Geometry check sheet. Reference: the model listing, model coordinates, mm. Coordinates: 2 decimals unless noted, no trailing zeros. Order: outer loops, then holes, each group sorted by start corner. A loop starts at its lowest first (then second) coordinate and runs counter-clockwise, first axis right, second up. Notation, with made-up numbers: M 20,85.5 L 70,85.5 A26 ccw 70,118.5 Z; hole C 63.5,70 d6. An arc over 180 degrees is marked long. One line per item, written item: value. Start each with the question number.
1) Go/stop test with flat-tipped pins: P1, Ø6.5, axis at x = -45, z = -30.5, coming from the +Y side; P2, Ø1.6, axis at x = 61, y = 3.5, coming from the +Z side; P3, Ø5, axis at x = 28, z = 3.5, coming from the +Y side; P4, Ø1.9, axis at x = -60, y = 3, coming from the -Z side. Record where each tip stops, or that it passes through.
2) Thickness scan on L1, parallel to Z at x = -9, y = 0.45; L2, parallel to Z at x = 52.5, y = 2.5; L3, parallel to Z at x = 48.5, y = 2.5. Record the ranges inside material, lowest first. Write a range as from..to.
3) Sectioned sample at A-A, the plane z = 23.5. State how many separate pieces and enclosed holes the cut face has, then the cut area to 3 significant figures.
4) Sectioned sample at B-B, the plane x = 20. Enter the section's corners in (y, z), then the cut area to 3 significant figures.
```python
from build123d import *

# Parameters (mm, degrees)
SKETCH1_W           = 131.727
SKETCH1_H           = 90.551
SKETCH1_R           = 3.5
BOSS_EXTRUDE1_DEPTH = 10
SKETCH3_W           = 10
SKETCH3_H           = 10
BOSS_EXTRUDE3_DEPTH = 10
SKETCH4_R           = 3.15
CUT_EXTRUDE2_DEPTH  = 87.564320205
FILLET2_R           = 2.5
FILLET3_R           = 4
SKETCH5_R           = 4.975
CUT_EXTRUDE3_DEPTH  = 9.5


with BuildPart() as part:
    # Sketch1 → Boss-Extrude1 (new body)
    with BuildSketch(Plane(origin=(0, 0, 0), x_dir=(1, 0, 0), z_dir=(0, 1, 0))):
        Rectangle(SKETCH1_W, SKETCH1_H)
        with Locations(Location((-45, 30.5, 0), (0, 0, 270))):
            Circle(SKETCH1_R, mode=Mode.SUBTRACT)
        with Locations(Location((-27, 30.5, 0), (0, 0, 270))):
            Circle(SKETCH1_R, mode=Mode.SUBTRACT)
        with Locations(Location((-9, 30.5, 0), (0, 0, 270))):
            Circle(SKETCH1_R, mode=Mode.SUBTRACT)
        with Locations(Location((9, 30.5, 0), (0, 0, 270))):
            Circle(SKETCH1_R, mode=Mode.SUBTRACT)
        with Locations(Location((27, 30.5, 0), (0, 0, 270))):
            Circle(SKETCH1_R, mode=Mode.SUBTRACT)
        with Locations(Location((45, 30.5, 0), (0, 0, 270))):
            Circle(SKETCH1_R, mode=Mode.SUBTRACT)
        with Locations(Location((-27, 12.5, 0), (0, 0, 270))):
            Circle(SKETCH1_R, mode=Mode.SUBTRACT)
        with Locations(Location((-9, 12.5, 0), (0, 0, 270))):
            Circle(SKETCH1_R, mode=Mode.SUBTRACT)
        with Locations(Location((9, 12.5, 0), (0, 0, 270))):
            Circle(SKETCH1_R, mode=Mode.SUBTRACT)
        with Locations(Location((27, 12.5, 0), (0, 0, 270))):
            Circle(SKETCH1_R, mode=Mode.SUBTRACT)
        with Locations(Location((45, 12.5, 0), (0, 0, 270))):
            Circle(SKETCH1_R, mode=Mode.SUBTRACT)
        with Locations(Location((-27, -5.5, 0), (0, 0, 270))):
            Circle(SKETCH1_R, mode=Mode.SUBTRACT)
        with Locations(Location((-9, -5.5, 0), (0, 0, 270))):
            Circle(SKETCH1_R, mode=Mode.SUBTRACT)
        with Locations(Location((9, -5.5, 0), (0, 0, 270))):
            Circle(SKETCH1_R, mode=Mode.SUBTRACT)
        with Locations(Location((27, -5.5, 0), (0, 0, 270))):
            Circle(SKETCH1_R, mode=Mode.SUBTRACT)
        with Locations(Location((45, -5.5, 0), (0, 0, 270))):
            Circle(SKETCH1_R, mode=Mode.SUBTRACT)
        with Locations(Location((-27, -23.5, 0), (0, 0, 270))):
            Circle(SKETCH1_R, mode=Mode.SUBTRACT)
        with Locations(Location((-9, -23.5, 0), (0, 0, 270))):
            Circle(SKETCH1_R, mode=Mode.SUBTRACT)
        with Locations(Location((9, -23.5, 0), (0, 0, 270))):
            Circle(SKETCH1_R, mode=Mode.SUBTRACT)
        with Locations(Location((27, -23.5, 0), (0, 0, 270))):
            Circle(SKETCH1_R, mode=Mode.SUBTRACT)
        with Locations(Location((45, -23.5, 0), (0, 0, 270))):
            Circle(SKETCH1_R, mode=Mode.SUBTRACT)
        with Locations(Location((-45, 12.5, 0), (0, 0, 270))):
            Circle(SKETCH1_R, mode=Mode.SUBTRACT)
        with Locations(Location((-45, -5.5, 0), (0, 0, 270))):
            Circle(SKETCH1_R, mode=Mode.SUBTRACT)
        with Locations(Location((-45, -23.5, 0), (0, 0, 270))):
            Circle(SKETCH1_R, mode=Mode.SUBTRACT)
    extrude(amount=BOSS_EXTRUDE1_DEPTH)

    # Sketch3 → Boss-Extrude3 (add)
    with BuildSketch(Plane.XZ):
        with Locations((52.3134, -50.2755)):
            Rectangle(SKETCH3_W, SKETCH3_H)
        with Locations((-50.47267, -50.2755)):
            Rectangle(SKETCH3_W, SKETCH3_H)
        with Locations((-50.47267, 50.2755)):
            Rectangle(SKETCH3_W, SKETCH3_H)
        with Locations((52.3134, 50.2755)):
            Rectangle(SKETCH3_W, SKETCH3_H)
    extrude(amount=-BOSS_EXTRUDE3_DEPTH)

    # Sketch4 → Cut-Extrude2 (cut, through all)
    with BuildSketch(Plane(origin=(0, 0, 0), x_dir=(-1, 0, 0), z_dir=(0, -1, 0))):
        with Locations(Location((-52.3134, -50.2755, 0), (0, 0, 90))):
            Circle(SKETCH4_R)
        with Locations(Location((50.47267, -50.2755, 0), (0, 0, 90))):
            Circle(SKETCH4_R)
        with Locations(Location((50.47267, 50.2755, 0), (0, 0, 90))):
            Circle(SKETCH4_R)
        with Locations(Location((-52.3134, 50.2755, 0), (0, 0, 90))):
            Circle(SKETCH4_R)
    extrude(amount=-CUT_EXTRUDE2_DEPTH, mode=Mode.SUBTRACT)

    # Fillet2
    fillet2_edges = [part.edges().sort_by_distance(p)[0] for p in [
        (47.3134, 5, 55.2755),
        (47.3134, 5, 45.2755),
        (57.3134, 5, 55.2755),
        (57.3134, 5, 45.2755),
        (-45.47267, 5, 55.2755),
        (-45.47267, 5, 45.2755),
        (-55.47267, 5, 55.2755),
        (-55.47267, 5, 45.2755),
        (-45.47267, 5, -45.2755),
        (-45.47267, 5, -55.2755),
        (-55.47267, 5, -45.2755),
        (-55.47267, 5, -55.2755),
        (47.3134, 5, -45.2755),
        (47.3134, 5, -55.2755),
        (57.3134, 5, -45.2755),
        (57.3134, 5, -55.2755),
    ]]
    fillet(fillet2_edges, radius=FILLET2_R)

    # Fillet3
    fillet3_edges = [part.edges().sort_by_distance(p)[0] for p in [
        (-65.8635, 5, -45.2755),
        (-65.8635, 5, 45.2755),
        (65.8635, 5, 45.2755),
        (65.8635, 5, -45.2755),
    ]]
    fillet(fillet3_edges, radius=FILLET3_R)

    # Sketch5 → Cut-Extrude3 (cut)
    with BuildSketch(Plane(origin=(0, 10, 0), x_dir=(1, 0, 0), z_dir=(0, 1, 0))):
        with Locations(Location((45, -23.5, 0), (0, 0, 270))):
            Circle(SKETCH5_R)
        with Locations(Location((27, -23.5, 0), (0, 0, 270))):
            Circle(SKETCH5_R)
        with Locations(Location((9, -23.5, 0), (0, 0, 270))):
            Circle(SKETCH5_R)
        with Locations(Location((-9, -23.5, 0), (0, 0, 270))):
            Circle(SKETCH5_R)
        with Locations(Location((-27, -23.5, 0), (0, 0, 270))):
            Circle(SKETCH5_R)
        with Locations(Location((-45, -23.5, 0), (0, 0, 270))):
            Circle(SKETCH5_R)
        with Locations(Location((45, -5.5, 0), (0, 0, 270))):
            Circle(SKETCH5_R)
        with Locations(Location((27, -5.5, 0), (0, 0, 270))):
            Circle(SKETCH5_R)
        with Locations(Location((9, -5.5, 0), (0, 0, 270))):
            Circle(SKETCH5_R)
        with Locations(Location((-9, -5.5, 0), (0, 0, 270))):
            Circle(SKETCH5_R)
        with Locations(Location((-27, -5.5, 0), (0, 0, 270))):
            Circle(SKETCH5_R)
        with Locations(Location((-45, -5.5, 0), (0, 0, 270))):
            Circle(SKETCH5_R)
        with Locations(Location((45, 12.5, 0), (0, 0, 270))):
            Circle(SKETCH5_R)
        with Locations(Location((27, 12.5, 0), (0, 0, 270))):
            Circle(SKETCH5_R)
        with Locations(Location((9, 12.5, 0), (0, 0, 270))):
            Circle(SKETCH5_R)
        with Locations(Location((-9, 12.5, 0), (0, 0, 270))):
            Circle(SKETCH5_R)
        with Locations(Location((-27, 12.5, 0), (0, 0, 270))):
            Circle(SKETCH5_R)
        with Locations(Location((-45, 12.5, 0), (0, 0, 270))):
            Circle(SKETCH5_R)
        with Locations(Location((45, 30.5, 0), (0, 0, 270))):
            Circle(SKETCH5_R)
        with Locations(Location((27, 30.5, 0), (0, 0, 270))):
            Circle(SKETCH5_R)
        with Locations(Location((9, 30.5, 0), (0, 0, 270))):
            Circle(SKETCH5_R)
        with Locations(Location((-9, 30.5, 0), (0, 0, 270))):
            Circle(SKETCH5_R)
        with Locations(Location((-27, 30.5, 0), (0, 0, 270))):
            Circle(SKETCH5_R)
        with Locations(Location((-45, 30.5, 0), (0, 0, 270))):
            Circle(SKETCH5_R)
    extrude(amount=-CUT_EXTRUDE3_DEPTH, mode=Mode.SUBTRACT)


solid = part.part
```
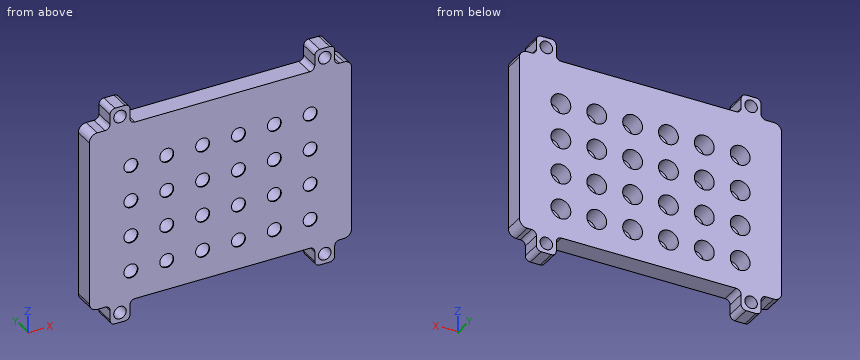
Final values:
1. P1: passes through
1. P2: stops at z = 45.28
1. P3: stops at y = 0.5
1. P4: stops at z = -45.28
2. L1: z = -45.28..-34, -27..-16, -9..2, 9..20, 27..45.28
2. L2: z = -55.28..-53.42, -47.13..47.13, 53.42..55.28
2. L3: z = -54.9..-34.04, -26.96..-16.04, -8.96..1.96, 9.04..19.96, 27.04..54.9
3. separate pieces: 7
3. enclosed holes: 0
3. area: 729 mm^2
4. outline: M 0,-45.28 L 10,-45.28 L 10,45.28 L 0,45.28 Z
4. area: 906 mm^2
